```python
from build123d import *

# Parameters (mm, degrees)
SKIZZE1_W                       = 50
SKIZZE1_H                       = 400
AUFSATZ_LINEAR_AUSTRAGEN1_DEPTH = 50
LINEARES_MUSTER1_COUNT          = 4
LINEARES_MUSTER1_PITCH          = 120


with BuildPart() as part:
    # Skizze1 → Aufsatz-Linear austragen1 (new body)
    with BuildSketch(Plane(origin=(0, 0, 0), x_dir=(1, 0, 0), z_dir=(0, 1, 0))):
        Rectangle(SKIZZE1_W, SKIZZE1_H)
    extrude(amount=AUFSATZ_LINEAR_AUSTRAGEN1_DEPTH)

    # Skizze2 → Ø9.5 (9.5) Durchmesser Bohrung1 (revolve, cut)
    with BuildSketch(Plane(origin=(0, 50, 180), x_dir=(0, 0, 1), z_dir=(1, 0, 0))):
        Polygon((0, 0), (0, 22.85408794), (4.75, 20), (4.75, 0), align=None)
    f_9_5_9_5_durchmesser_bohrung1 = revolve(axis=Axis((0, 56.35, 180), (0, -1, 0)), mode=Mode.SUBTRACT)

    # Lineares Muster1: Ø9.5 (9.5) Durchmesser Bohrung1 ×4
    with Locations(*[(0, 0, -i * LINEARES_MUSTER1_PITCH) for i in range(1, LINEARES_MUSTER1_COUNT)]):
        add(f_9_5_9_5_durchmesser_bohrung1, mode=Mode.SUBTRACT)


solid = part.part
```
Part model, mm, in its own coordinate system. A direction names the side the tool comes from. Round coordinates to 2 decimals unless told otherwise and drop trailing zeros. Return JSON: item names as keys, results as strings. Group by question number.
Q1. Mould opens along X. For faces 1 (the flat face through (25, 25, 3)), 2 (the cylindrical face through (-0.209, 40.14, -64.745)), 3 (the flat face through (0, 25, -200)) say: pulls with the +X half, pulls with the -X half, needs draft (parallel to the pull), parting line crosses it, or undercut.
Q2. Pin check, flat tip, straight feed: pin 1 (7.5 mm diameter, centred on x = 0, z = 60, fed in from +Y). Stop position of the tip, or through.
Q3. Probe L1, parallel to Z at x = 0, y = 38; L2, parallel to X at y = 44.25, z = -180; L3, parallel to Z at x = -2.5, y = 41.5. List the from-to ranges inside material, lowest first. Write a range as [from, to].
Q4. Which spindle directions (+Z, -Z, +X, -X, +Y, -Y) get a long thin tool onto all of the face, cutting with end or side? Do faces 4 (the flat face through (0, 50, -3)), 5 (the cylindrical face through (-0.209, 40.14, -184.745)). Say none if no direction does.
Answer:
{
 "1": {"face 1": "pulls with the +X half", "face 2": "undercut", "face 3": "needs draft"},
 "2": {"pin 1": "y = 29.4"},
 "3": {"L1": "[-200, -184.75], [-175.25, -64.75], [-55.25, 55.25], [64.75, 175.25], [184.75, 200]", "L2": "[-25, -4.75], [4.75, 25]", "L3": "[-200, -184.04], [-175.96, -64.04], [-55.96, 55.96], [64.04, 175.96], [184.04, 200]"},
 "4": {"face 4": "+Z, -Z, +X, -X, +Y", "face 5": "+Y"}
}
